Geometry check sheet. Reference: the model listing, model coordinates, mm. A direction names the side the tool comes from. Round coordinates to 2 decimals unless told otherwise and drop trailing zeros. Order: outer loops, then holes, each group sorted by start corner. A loop starts at its lowest first (then second) coordinate and runs counter-clockwise, first axis right, second up. Notation, with made-up numbers: (27.5, 12) -> (59.5, 12) arc R34 cw to (59.5, 49) -> close; hole circle Ø3 at (42.5, 52). An arc over 180 degrees is marked (long way). Answer as a JSON object with one key per item and string values. Group by question number.
from build123d import *

# Parameters (mm, degrees)
BOSS_EXTRUDE1_DEPTH = 6
HOLE2_D             = 4
HOLE2_DEPTH         = 3
HOLE2_CBORE_D       = 5
HOLE2_CBORE_DEPTH   = 0.8
HOLE2_TIP           = 1.201721238
HOLE3_D             = 4
HOLE3_DEPTH         = 18
HOLE3_CBORE_D       = 5
HOLE3_CBORE_DEPTH   = 0.8
HOLE3_TIP           = 1.201721238
CUT_EXTRUDE1_START  = -0.8
CUT_EXTRUDE1_DEPTH  = 0.8
CUT_EXTRUDE2_START  = -0.8
SKETCH12_R          = 2.5
CUT_EXTRUDE2_DEPTH  = 0.8
SKETCH14_R          = 2.35
CUT_EXTRUDE3_DEPTH  = 0.8
CHAMFER1_SIZE       = 1.5
FILLET1_R           = 3


with BuildPart() as part:
    # Sketch1 → Boss-Extrude1 (new, symmetric)
    with BuildSketch(Plane.XY):
        Polygon((0, 7.5), (0, -7.5), (18, -7.5), (18, -4.5), (3, -4.5), (3, 7.5), align=None)
    extrude(amount=BOSS_EXTRUDE1_DEPTH, both=True)

    # Hole2
    with Locations(Plane(origin=(0, -4.5, 0), x_dir=(1, 0, 0), z_dir=(0, 1, 0))):
        with Locations((15, 3), (9, 3), (9, -3), (15, -3)):
            CounterBoreHole(HOLE2_D / 2, HOLE2_CBORE_D / 2, HOLE2_CBORE_DEPTH, depth=HOLE2_DEPTH)
            with Locations((0, 0, -(HOLE2_DEPTH + HOLE2_TIP / 2))):  # 118° drill point
                Cone(0, HOLE2_D / 2, HOLE2_TIP, mode=Mode.SUBTRACT)

    # Hole3
    with Locations(Plane.ZY):
        with Locations((3, -1.5), (-3, -1.5), (3, 4.5), (-3, 4.5)):
            CounterBoreHole(HOLE3_D / 2, HOLE3_CBORE_D / 2, HOLE3_CBORE_DEPTH, depth=HOLE3_DEPTH)
            with Locations((0, 0, -(HOLE3_DEPTH + HOLE3_TIP / 2))):  # 118° drill point
                Cone(0, HOLE3_D / 2, HOLE3_TIP, mode=Mode.SUBTRACT)

    # Sketch11 → Cut-Extrude1 (cut)
    with BuildSketch(Plane(origin=(3, 0, 0), x_dir=(0, 0, -1), z_dir=(1, 0, 0)).offset(CUT_EXTRUDE1_START)):
        with BuildLine():
            Line((5.5, -1.5), (5.5, 7.5))
            Line((5.5, 7.5), (0.5, 7.5))
            Line((0.5, 7.5), (0.5, -1.5))
            ThreePointArc((0.5, -1.5), (3, -4), (5.5, -1.5))
        make_face()
    cut_extrude1 = extrude(amount=CUT_EXTRUDE1_DEPTH, mode=Mode.SUBTRACT)

    # Sketch12 → Cut-Extrude2 (cut)
    with BuildSketch(Plane(origin=(0, -7.5, 0), x_dir=(-1, 0, 0), z_dir=(0, -1, 0)).offset(CUT_EXTRUDE2_START)):
        with Locations(Location((-9, 3, 0), (0, 0, 270))):
            Circle(SKETCH12_R)
        with Locations(Location((-15, 3, 0), (0, 0, 270))):
            Circle(SKETCH12_R)
        with BuildLine():
            Line((-3, 0.5), (0, 0.5))
            Line((0, 0.5), (0, 5.5))
            Line((0, 5.5), (-3, 5.5))
            ThreePointArc((-3, 5.5), (-5.5, 3), (-3, 0.5))
        make_face()
    cut_extrude2 = extrude(amount=CUT_EXTRUDE2_DEPTH, mode=Mode.SUBTRACT)

    # Sketch14 → Cut-Extrude3 (cut)
    with BuildSketch(Plane.ZY):
        with Locations((-3, -7.5)):
            Circle(SKETCH14_R)
    cut_extrude3 = extrude(amount=-CUT_EXTRUDE3_DEPTH, mode=Mode.SUBTRACT)

    # Mirror1: Cut-Extrude1, Cut-Extrude2, Cut-Extrude3 across plane
    add(cut_extrude1.mirror(Plane.XY), mode=Mode.SUBTRACT)
    add(cut_extrude2.mirror(Plane.XY), mode=Mode.SUBTRACT)
    add(cut_extrude3.mirror(Plane.XY), mode=Mode.SUBTRACT)

    # Chamfer1
    # the kernel refuses this chamfer: 1.5 mm, written as the material it takes off along each edge
    with BuildSketch(Plane(origin=(0, -7.5, 1.642475518), x_dir=(-0.027495876610586376, 0.9996219169112968, 0), z_dir=(0, 0, 1)), Plane(origin=(0, -7.5, -9.857524482), x_dir=(-0.027495876610586376, 0.9996219169112968, 0), z_dir=(0, 0, 1))) as chamfer1_piece_1:
        Polygon((CHAMFER1_SIZE * 0.999621916911, -CHAMFER1_SIZE * 0.0274958766106), (-CHAMFER1_SIZE * 0.0274958766106, -CHAMFER1_SIZE * 0.999621916911), (0, 0), align=None)
    extrude(amount=8.215048964, mode=Mode.SUBTRACT)
    with BuildSketch(Plane(origin=(0, -7.5, -4.357524482), x_dir=(-0.027495876610586376, 0.9996219169112968, 0), z_dir=(0, 0, 1))) as chamfer1_piece_2:
        Polygon((CHAMFER1_SIZE * 0.999621916911, -CHAMFER1_SIZE * 0.0274958766106), (-CHAMFER1_SIZE * 0.0274958766106, -CHAMFER1_SIZE * 0.999621916911), (0, 0), align=None)
    extrude(amount=8.715048964, mode=Mode.SUBTRACT)

    # Fillet1
    fillet1_edges = [part.edges().sort_by_distance(p)[0] for p in [
        (18, -6, 6),
        (18, -6, -6),
        (1.5, 7.5, 6),
        (1.5, 7.5, -6),
    ]]
    fillet(fillet1_edges, radius=FILLET1_R)


solid = part.part
Item 1: Sectioned sample at D-D, the plane z = 4. Count the separate pieces of the cut face and the enclosed holes in it, then the cut area to 3 significant figures.
Item 2: Thickness scan on L1, parallel to Z at x = 9, y = -4.75; L2, parallel to X at y = -5.25, z = 2.5; L3, parallel to Z at x = 16.25, y = -5.5. Record the ranges inside material, lowest first.
Item 3: Sectioned sample at A-A, the plane x = 9. Enter the section's corners in (y, z), then the cut area to 3 significant figures.
Item 4: Sectioned sample at B-B, the plane y = 4. Enter the section's corners in (x, z).
Item 5: Depth check by flat-ended pin: pin 1 Ø5.5 at (x, z) = (14, -3) entering from +Y; pin 2 Ø4 at (y, z) = (0.5, 3) entering from +X; pin 3 Ø1.2 at (y, z) = (-6, 3.5) entering from -X. Enter the tip coordinate at first touch or a pass-through.
Item 6: Mould release check, pull along Y, two halves, no side actions. Record for faces 6 (the flat face through (6, -5, 6)), 7 (the flat face through (13, -6.7, -4)), 8 (the cylindrical face through (1.51, 2.548, 3.434)): pulls with the +Y half, pulls with the -Y half, needs draft (parallel to the pull), parting line crosses it, or undercut.
Item 7: Sectioned sample at C-C, the plane y = 1.75. Enter the section's corners in (x, z).
Item 8: Set-up check for faces 1 (the flat face through (2, -7, 5.5)), 2 (the cylindrical face through (12.5, -4.9, 2.9)), 3 (the flat face through (2.2, 2, 3)), 4 (the flat face through (3, 0, 0)), 5 (the flat face through (7, -6.7, -4)): record each of +Z, -Z, +X, -X, +Y, -Y from which the full face is reachable in a straight line by a thin tool's end or side.
Result:
{
 "1": {"separate pieces": "5", "enclosed holes": "0", "area": "33.4 mm2"},
 "2": {"L1": "z = -6 to -5.5, -0.5 to 0.5, 5.5 to 6", "L2": "x = 0.8 to 6.55, 11.45 to 12.55, 17.45 to 18", "L3": "z = -5.73 to -4.56, -1.44 to 1.44, 4.56 to 5.73"},
 "3": {"outline": "(-7.5, -6) -> (-4.5, -6) -> (-4.5, -5.5) -> (-5.3, -5.5) -> (-5.3, -5) -> (-6.7, -5) -> (-6.7, -5.5) -> (-7.5, -5.5) -> close; (-7.5, -0.5) -> (-6.7, -0.5) -> (-6.7, -1) -> (-5.3, -1) -> (-5.3, -0.5) -> (-4.5, -0.5) -> (-4.5, 0.5) -> (-5.3, 0.5) -> (-5.3, 1) -> (-6.7, 1) -> (-6.7, 0.5) -> (-7.5, 0.5) -> close; (-7.5, 5.5) -> (-6.7, 5.5) -> (-6.7, 5) -> (-5.3, 5) -> (-5.3, 5.5) -> (-4.5, 5.5) -> (-4.5, 6) -> (-7.5, 6) -> close", "area": "8.80 mm2"},
 "4": {"outline": "(0, -6) -> (3, -6) -> (3, -5.5) -> (2.2, -5.5) -> (2.2, -4.94) -> (0.8, -4.94) -> (0.8, -5.45) -> (0, -5.45) -> close; (0, -0.55) -> (0.8, -0.55) -> (0.8, -1.06) -> (2.2, -1.06) -> (2.2, -0.5) -> (3, -0.5) -> (3, 0.5) -> (2.2, 0.5) -> (2.2, 1.06) -> (0.8, 1.06) -> (0.8, 0.55) -> (0, 0.55) -> close; (0, 5.45) -> (0.8, 5.45) -> (0.8, 4.94) -> (2.2, 4.94) -> (2.2, 5.5) -> (3, 5.5) -> (3, 6) -> (0, 6) -> close"},
 "5": {"pin 1": "stops at y = -4.5", "pin 2": "stops at x = 2.2", "pin 3": "stops at x = 0.8"},
 "6": {"face 6": "needs draft", "face 7": "pulls with the -Y half", "face 8": "undercut"},
 "7": {"outline": "(0, -6) -> (3, -6) -> (3, -5.5) -> (2.2, -5.5) -> (2.2, -0.5) -> (3, -0.5) -> (3, 0.5) -> (2.2, 0.5) -> (2.2, 5.5) -> (3, 5.5) -> (3, 6) -> (0, 6) -> close"},
 "8": {"face 1": "-X, -Y", "face 2": "+Y", "face 3": "+X, +Y", "face 4": "+Z, -Z, +X, +Y", "face 5": "-Y"}
}
